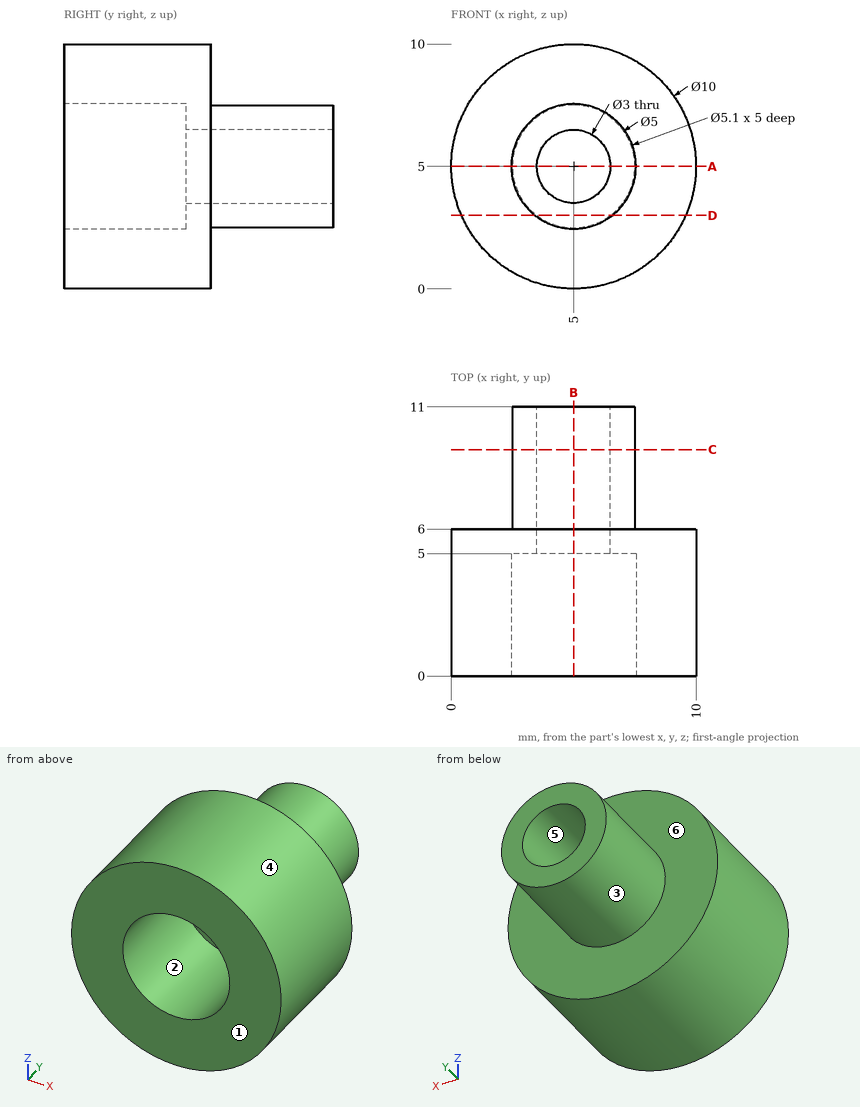
Geometry: see drawing. Coordinates: mm, zero at the bounding-box minimum. A direction names the side the tool comes from. Round coordinates to 2 decimals unless told otherwise and drop trailing zeros. Write each loop counter-clockwise with the first axis right and the second up, starting at its lowest first coordinate (ties: lowest second). Pieces come first, ordered by that corner, then holes. Notation, with made-up numbers: M 46.25,76 L 72.25,76 A8 cw 72.25,80 Z; hole C 76,5.5 d7. An arc over 180 degrees is marked long. Answer as a JSON object with one key per item and string values. Group by question number.
(1) Ray query, line 1 (X direction, y = 3, z = 5); line 2 (Z direction, x = 3, y = 9.5); line 3 (X direction, y = 8.25, z = 5). Return the intervals inside material, ascending. Write a range as [from, to].
(2) Section query D-D on z = 3. Output: boundary loops of the cut face in (x, y).
(3) Section query B-B on x = 5. Output: boundary loops of the cut face in (y, z), then the cut area to 3 significant figures.
(4) Section query C-C on y = 9.25. Output: boundary loops of the cut face in (x, z).
(5) Section query A-A on z = 5. Output: boundary loops of the cut face in (x, y), then the cut area to 3 significant figures.
(6) Mould query, pull axis Z, two halves, no side actions, for the marked faces 4, 5 and 6. Classes: +Z half, -Z half, draft (parallel to the pull), parting line (faces both ways), or undercut.
(7) Reachability of the marked faces 1, 2 and 3 from +Z, -Z, +X, -X, +Y, -Y: full face, straight path, thin tool, end or side. Return the list, or none.
(8) First-contact query: pin 1 (1.5 mm diameter, centred on x = 4.5, z = 5.5, fed in from -Y); pin 2 (2 mm diameter, centred on y = 2, z = 8.5, fed in from +X); pin 3 (1.5 mm diameter, centred on x = 4, z = 3, fed in from -Y); pin 4 (4.5 mm diameter, centred on x = 5, z = 5, fed in from -Y). Flat tips, straight axial feed; report the tip coordinate or a pass-through.
Computed values:
{
 "1": {"line 1": "[0, 2.45], [7.55, 10]", "line 2": "[3.5, 6.5]", "line 3": "[2.5, 3.5], [6.5, 7.5]"},
 "2": {"outline": "M 0.42,0 L 3.42,0 L 3.42,5 L 6.58,5 L 6.58,0 L 9.58,0 L 9.58,6 L 6.5,6 L 6.5,11 L 3.5,11 L 3.5,6 L 0.42,6 Z"},
 "3": {"outline": "M 0,0 L 6,0 L 6,2.5 L 11,2.5 L 11,3.5 L 5,3.5 L 5,2.45 L 0,2.45 Z; M 0,7.55 L 5,7.55 L 5,6.5 L 11,6.5 L 11,7.5 L 6,7.5 L 6,10 L 0,10 Z", "area": "41.5 mm^2"},
 "4": {"outline": "C 5,5 d5; hole C 5,5 d3"},
 "5": {"outline": "M 0,0 L 2.45,0 L 2.45,5 L 3.5,5 L 3.5,11 L 2.5,11 L 2.5,6 L 0,6 Z; M 6.5,5 L 7.55,5 L 7.55,0 L 10,0 L 10,6 L 7.5,6 L 7.5,11 L 6.5,11 Z", "area": "41.5 mm^2"},
 "6": {"face 4": "parting line", "face 5": "undercut", "face 6": "draft"},
 "7": {"face 1": "+Z, -Z, +X, -X, -Y", "face 2": "-Y", "face 3": "+Y"},
 "8": {"pin 1": "through", "pin 2": "x = 9.33", "pin 3": "y = 0", "pin 4": "y = 5"}
}
